Source: CAD feature listing. Evaluate the final solid. Frame: model axes, mm. A direction names the side the tool comes from. Coordinates: 2 decimals unless noted, no trailing zeros. Order: outer loops, then holes, each group sorted by start corner. A loop starts at its lowest first (then second) coordinate and runs counter-clockwise, first axis right, second up.
```python
from build123d import *

# Parameters (mm, degrees)
BOSS_EXTRUDE1_DEPTH = 10
SKETCH2_R           = 1.5
CUT_EXTRUDE1_DEPTH  = 10
SKETCH4_R           = 1.5
CUT_EXTRUDE2_DEPTH  = 10


with BuildPart() as part:
    # Sketch1 → Boss-Extrude1 (new body)
    with BuildSketch(Plane(origin=(0, 0, 0), x_dir=(0, 0, -1), z_dir=(1, 0, 0))):
        Polygon((0, 0), (0, 15), (11.490666647, 24.641814145), (12.776241866, 23.109725259), (2, 14.067384684), (2, 0), align=None)
    extrude(amount=BOSS_EXTRUDE1_DEPTH)

    # Sketch2 → Cut-Extrude1 (cut)
    with BuildSketch(Plane.XY):
        with Locations((5, 5)):
            Circle(SKETCH2_R)
    extrude(amount=-CUT_EXTRUDE1_DEPTH, mode=Mode.SUBTRACT)

    # Sketch4 → Cut-Extrude2 (cut)
    with BuildSketch(Plane(origin=(0, 8.802361333, 7.386058148), x_dir=(1, 0, 0), z_dir=(0, 0.7660444431189788, 0.6427876096865384))):
        with Locations(Location((5, 19.641814145, 0), (0, 0, 270))):
            Circle(SKETCH4_R)
    extrude(amount=-CUT_EXTRUDE2_DEPTH, mode=Mode.SUBTRACT)


solid = part.part
```
1. Contact query for flat-ended pins moving along their axis: P1, Ø3, axis at x = 6.5, y = 8.5, coming from the -Z side; P2, Ø6, axis at x = 5, z = -10, coming from the -Y side; P3, Ø5, axis at x = 2.5, z = -5, coming from the -Y side; P4, Ø2.5, axis at x = 5, y = 5, coming from the +Z side (3 decimals). Output: stop coordinate, or through.
2. Section query B-B, the plane x = 4.75. Output: boundary loops of the cut face in (y, z), plus the area to 3 significant figures.
3. Draft query along Z for faces 1 (the cylindrical face through (6.386, 4.425, -0.986)), 2 (the flat face through (4.93, 19.75, -5.66)), 3 (the cylindrical face through (4.43, 19.78, -7.23)), 4 (the flat face through (4.93, 18.65, -7.46)). Return one class per face: +Z half, -Z half, draft (parallel to the pull), parting line (faces both ways), or undercut.
4. Section query A-A, the plane y = 5. Output: boundary loops of the cut face in (x, z).
5. Section query D-D, the plane x = 3.25. Output: boundary loops of the cut face in (y, z), plus the area to 3 significant figures.
6. Access query for faces 5 (the flat face through (5, 7, -2)), 6 (the flat face through (0, 15.1, -2.6)). Directions: +Z, -Z, +X, -X, +Y, -Y. A direction counts if a zero-diameter tool reaches every point of the face in a straight line with its end or side. Return the directions, or none.
7. Section query C-C, the plane z = -1.5. Output: boundary loops of the cut face in (x, y).
8. Material intervals for line 1 along Z through (x, y) = (3, 6.25); line 2 along Y through (x, z) = (5, -0.95); line 3 along Z through (x, y) = (8, 16), sorted ascending.
Answer key:
1. P1: stops at z = -2
1. P2: stops at y = 18.26
1. P3: stops at y = 14.49
1. P4: passes through
2. outline: (0, -2) - (3.52, -2) - (3.52, 0) - (0, 0) - close; (6.48, -2) - (14.07, -2) - (18.95, -7.81) - (20.48, -6.53) - (15, 0) - (6.48, 0) - close; (20.85, -10.08) - (23.11, -12.78) - (24.64, -11.49) - (22.38, -8.79) - close
2. area: 46.3 mm2
3. face 1: draft
3. face 2: +Z half
3. face 3: undercut
3. face 4: -Z half
4. outline: (0, -2) - (3.5, -2) - (3.5, 0) - (0, 0) - close; (6.5, -2) - (10, -2) - (10, 0) - (6.5, 0) - close
5. outline: (0, -2) - (14.07, -2) - (23.11, -12.78) - (24.64, -11.49) - (15, 0) - (0, 0) - close
5. area: 58.1 mm2
6. face 5: -Z, +X, -X, -Y
6. face 6: +Z, -Z, -X, +Y, -Y
7. outline: (0, 0) - (10, 0) - (10, 16.26) - (0, 16.26) - close; hole circle Ø3 at (5, 5)
8. line 1: z = -2 to 0
8. line 2: y = 0 to 3.5, 6.5 to 15.8
8. line 3: z = -4.3 to -1.19
